The model under review builds one solid part; all positions refer to its coordinate system, in mm. A direction names the side the tool comes from. Round coordinates to 2 decimals unless told otherwise and drop trailing zeros. Write each loop counter-clockwise with the first axis right and the second up, starting at its lowest first coordinate (ties: lowest second). Pieces come first, ordered by that corner, then holes.
Item 1: Add section A-A (z = 10). Give the boundary of the cut face in (x, y), plus the area to 3 significant figures.
Item 2: Draft analysis for pull direction Y (two halves, no side actions). For faces 4 (the face through (-14.985, 0.66, 32.392)), 5 (the face through (19.334, 2.539, 16.479)), 6 (the face through (-19, 6, 12)), state which applies: +Y half, -Y half, draft (parallel to the pull), parting line (faces both ways), or undercut.
Item 3: Add section B-B (z = 20). Give the boundary of the cut face in (x, y).
Item 4: To check wall thickness, follow L1, parallel to Z at x = -21, y = 7; L2, parallel to Y at x = 0, z = 39; L3, parallel to Z at x = 9.5, y = -15.5. State the ranges of each line that lie inside material, in increasing order.
Item 5: Clearance check with flat-ended pins moving along their axes: pin 1 Ø4 at (x, y) = (13, 17.5) entering from +Z; pin 2 Ø6 at (x, z) = (14.5, 50) entering from +Y; pin 3 Ø1 at (y, z) = (-3, 26.5) entering from -X. State where each tip first meets the part, or that it passes through.
Item 6: Machinability: for faces 1 (the face through (-19, -6, 15)), 2 (the face through (-24.9, 5.5, 7.5)), 3 (the face through (-17, -6, 27)), which of the approach directions +Z, -Z, +X, -X, +Y, -Y give a long, thin tool a straight path to every point of the face, cutting with its end or side? Answer none if there is none.
```python
from build123d import *

# Parameters (mm, degrees)
F0_R     = 17.5
F1_DEPTH = 60
F2_R     = 15
F3_DEPTH = 56


with BuildPart() as f1:
    # F0 (on Top) → F1 (new body)
    with BuildSketch(Plane.XY):
        Circle(F0_R)
    extrude(amount=F1_DEPTH)

    # F2 (on face) → F3 (cut)
    with BuildSketch(Plane.XY.offset(60)):
        Circle(F2_R)
    extrude(amount=-F3_DEPTH, mode=Mode.SUBTRACT)

    # F4 (on Right) → F5 (revolve)
    with BuildSketch(Plane.YZ):
        Polygon((-25.5, 3), (-25.5, 0), (-17.5, 0), (-17.5, 27), (-25.5, 27), (-25.5, 24), (-19.5, 24), (-19.5, 21), (-25.5, 21), (-25.5, 18), (-19.5, 18), (-19.5, 15), (-25.5, 15), (-25.5, 12), (-19.5, 12), (-19.5, 9), (-25.5, 9), (-25.5, 6), (-19.5, 6), (-19.5, 3), align=None)
    revolve(axis=Axis((0, 0, 13.5), (0, 0, 1)))


solid = f1.part
```
Numbers:
1. outline: circle Ø39 at (0, 0); hole circle Ø30 at (0, 0)
1. area: 488 mm2
2. face 4: undercut
2. face 5: parting line
2. face 6: draft
3. outline: circle Ø51 at (0, 0); hole circle Ø30 at (0, 0)
4. L1: z = 0 to 3, 6 to 9, 12 to 15, 18 to 21, 24 to 27
4. L2: y = -17.5 to -15, 15 to 17.5
4. L3: z = 0 to 27
5. pin 1: stops at z = 27
5. pin 2: stops at y = 13.19
5. pin 3: stops at x = -25.38
6. face 1: none
6. face 2: +Z, -Z
6. face 3: +Z
